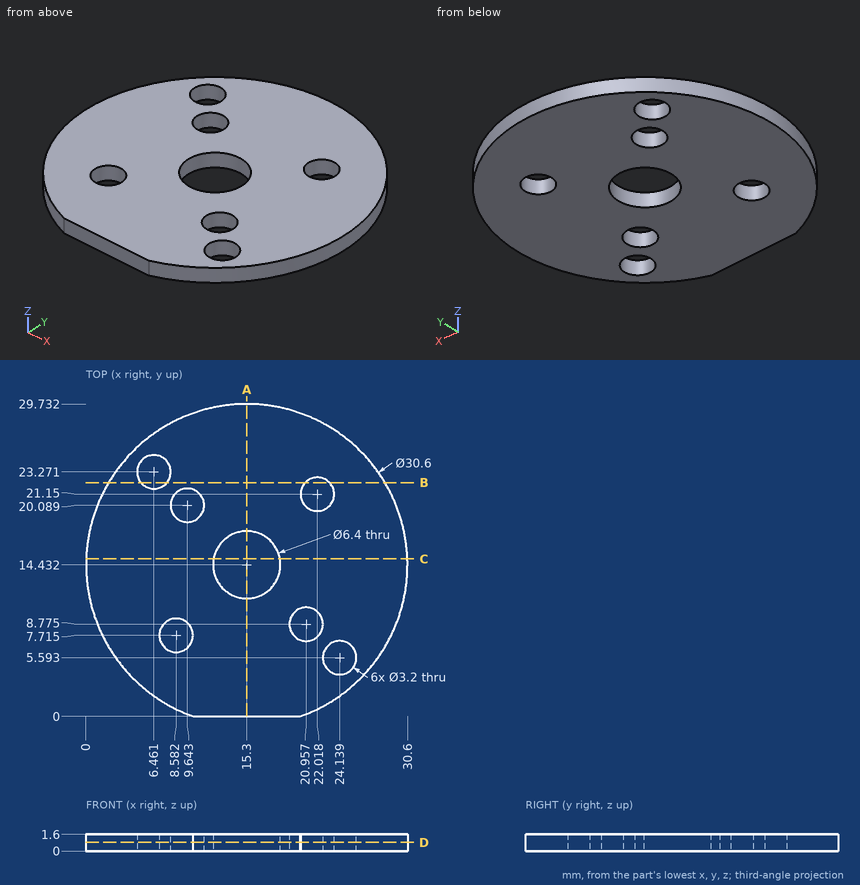
Job drawing, mm, ordinate dimensions from the low corner. One solid piece. Give positions to 0.01 mm unless a question says otherwise; leave off trailing zeros. Loops run counter-clockwise (first coordinate to the right, second up) from the corner with the lowest first, then second, coordinate; pieces in that order, holes last. Notation, with made-up numbers: (88.5, 44) -> (102.5, 44) arc R22 ccw to (102.5, 61) -> close; hole circle Ø11 at (-17.75, 31). An arc over 180 degrees is marked (long way). Use a Markdown table: item, result. Add a question column.
(1) Slice it at D-D on z = 0.85. Give the number of separate pieces and of enclosed holes in the cut face, and give its area (3 significant figures).
(2) Slice it at C-C on y = 15. List the corners of the cut face in (x, z).
(3) Wall check: line 1 along Y through (x, z) = (15.3, 1.15); line 2 along X through (y, z) = (8.5, 1.5) (1 decimal); line 3 along X through (y, z) = (8, 0.6) (1 decimal). Give the ranges that are in metal, low to high.
(4) Slice it at A-A on x = 15.3. List the corners of the cut face in (y, z).
(5) Slice it at B-B on y = 22.25. List the corners of the cut face in (x, z).
Filled sheet:
| question | item | result |
|---|---|---|
| 1 | separate pieces | 1 |
| 1 | enclosed holes | 7 |
| 1 | area | 649 mm2 |
| 2 | outline | (0.01, 0) -> (12.15, 0) -> (12.15, 1.6) -> (0.01, 1.6) -> close; (18.45, 0) -> (30.59, 0) -> (30.59, 1.6) -> (18.45, 1.6) -> close |
| 3 | line 1 | 0 to 11.23, 17.63 to 29.73 |
| 3 | line 2 | 1.2 to 7.2, 10 to 19.4, 22.5 to 29.4 |
| 3 | line 3 | 1.4 to 7, 10.2 to 19.6, 22.4 to 29.2 |
| 4 | outline | (0, 0) -> (11.23, 0) -> (11.23, 1.6) -> (0, 1.6) -> close; (17.63, 0) -> (29.73, 0) -> (29.73, 1.6) -> (17.63, 1.6) -> close |
| 5 | outline | (2.15, 0) -> (5.23, 0) -> (5.23, 1.6) -> (2.15, 1.6) -> close; (7.69, 0) -> (20.86, 0) -> (20.86, 1.6) -> (7.69, 1.6) -> close; (23.18, 0) -> (28.45, 0) -> (28.45, 1.6) -> (23.18, 1.6) -> close |
